Answer from the drawing. Dimensions are ordinates in mm from the lowest x, y and z of the part. A direction names the side the tool comes from. Give positions to 0.01 mm unless a question says otherwise; leave off trailing zeros. Loops run counter-clockwise (first coordinate to the right, second up) from the corner with the lowest first, then second, coordinate; pieces in that order, holes last. Notation, with made-up numbers: (63, -32) - (116, -32) arc R29 ccw to (116, 2) - close; hole circle Ø6 at (9, 55). An arc over 180 degrees is marked (long way). Put each result on its own line as item: value. Start each with the question number.
1. Given pin 1 Ø1 at (y, z) = (2.5, 2) entering from -X; pin 2 Ø1.7 at (y, z) = (3, 2.5) entering from +X, each flat-ended and moving along its own axis, determine where each tip first touches the part or whether it passes through.
2. Consider L1, parallel to X at y = 5.75, z = 5.25 (1 decimal); L2, parallel to X at y = 4, z = 6 (1 decimal); L3, parallel to Y at x = 3.5, z = 5 (1 decimal). Determine where each line is inside the solid, lowest interval first. Write a range as from..to.
3. A cutting plane is placed at C-C, the plane z = 1. Count the separate pieces of the cut face and the enclosed holes in it, plus the area to 3 significant figures.
4. For the marked faces 1 and 2, determine the directions among +Z, -Z, +X, -X, +Y, -Y from which every point of the face is accessible in a straight line to the end or side of a thin tool.
5. A cutting plane is placed at B-B, the plane y = 2.5. Determine the outline of the cut face in (x, z).
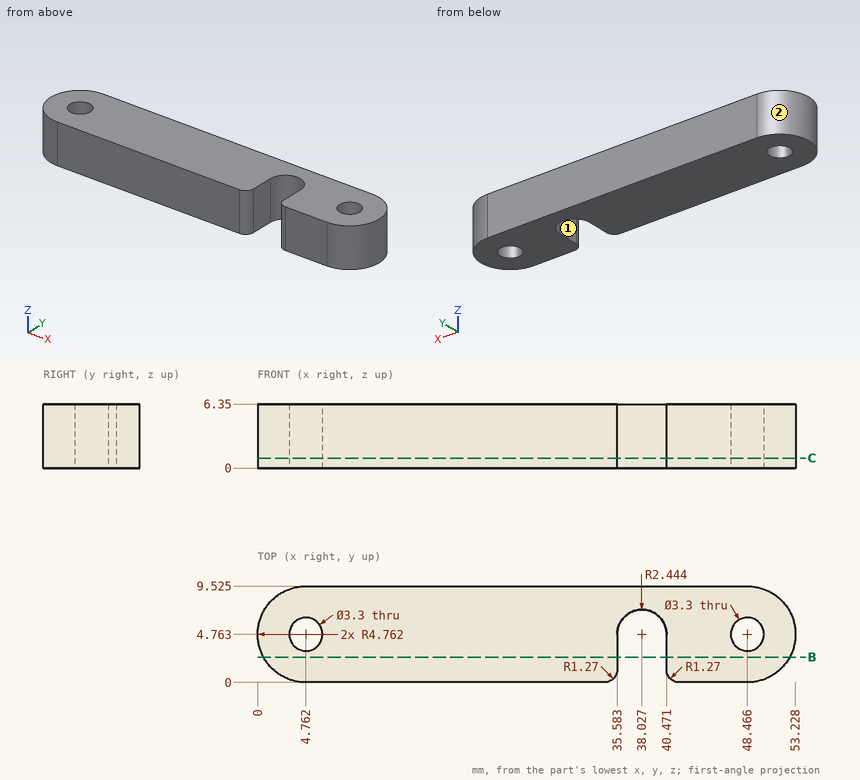
Return value:
1. pin 1: stops at x = 0.34
1. pin 2: stops at x = 53.14
2. L1: x = 0.1..3.4, 6.1..35.8, 40.3..47.1, 49.8..53.1
2. L2: x = 0.1..3.3, 6.2..35.6, 40.5..47, 49.9..53.2
2. L3: y = 0.2..3.7, 5.8..9.4
3. separate pieces: 1
3. enclosed holes: 2
3. area: 437 mm2
4. face 1: +Z, -Z, -Y
4. face 2: +Z, -Z, -X
5. outline: (0.57, 0) - (35.58, 0) - (35.58, 6.35) - (0.57, 6.35) - close; (40.47, 0) - (52.66, 0) - (52.66, 6.35) - (40.47, 6.35) - close
